Read the model definition and answer for the solid it produces. Units are mm, in the model's axes. Coordinates: 2 decimals unless noted, no trailing zeros. Order: outer loops, then holes, each group sorted by start corner. A loop starts at its lowest first (then second) coordinate and runs counter-clockwise, first axis right, second up. Notation, with made-up numbers: M 66.5,-6.5 L 112.5,-6.5 A15 cw 112.5,15.5 Z; hole C -20.75,14.5 d6. An arc over 180 degrees is marked long. Write each question's results on one line, items separated by ' | '.
```python
from build123d import *

# Parameters (mm, degrees)
SKETCH1_W           = 10
SKETCH1_H           = 24.4
SKETCH1_R           = 3
BOSS_EXTRUDE1_DEPTH = 10
FILLET1_R           = 2


with BuildPart() as part:
    # Sketch1 → Boss-Extrude1 (new body)
    with BuildSketch(Plane(origin=(0, 0, 0), x_dir=(1, 0, 0), z_dir=(0, 1, 0))):
        Rectangle(SKETCH1_W, SKETCH1_H)
        with Locations(Location((0, 0, 0), (0, 0, 270))):
            Circle(SKETCH1_R, mode=Mode.SUBTRACT)
    extrude(amount=BOSS_EXTRUDE1_DEPTH)

    # Fillet1
    fillet1_edges = [part.edges().sort_by_distance(p)[0] for p in [
        (-5, 10, 0),
        (5, 10, 0),
    ]]
    fillet(fillet1_edges, radius=FILLET1_R - 0.0001)  # a hair under: the kernel refuses the full size


solid = part.part
```
(1) The mould has two halves that part along X. Classify faces 1 (the cylindrical face through (4.43, 9.4, -0.17)), 2 (the cylindrical face through (0.9, 4.93, 2.86)), 3 (the cylindrical face through (-4.43, 9.4, -0.17)), 4 (the flat face through (-1, 10, -3)): pulls with the +X half, pulls with the -X half, needs draft (parallel to the pull), parting line crosses it, or undercut.
Conclusion:
face 1: pulls with the +X half | face 2: undercut | face 3: pulls with the -X half | face 4: needs draft
(2) Given pin 1 (1.5 mm diameter, centred on x = 0.5, z = 7, fed in from -Y); pin 2 (1.5 mm diameter, centred on x = -1, z = 0.5, fed in from -Y), each flat-ended and moving along its own axis, determine where each tip first touches the part or whether it passes through.
Conclusion:
pin 1: y = 0 | pin 2: through
(3) Straight lines are drawn through the part: line 1 (X direction, y = 4.75, z = 0); line 2 (Z direction, x = 0.75, y = 7.5); line 3 (X direction, y = 7, z = -0.75). For each, find the intervals that lie inside material, in ascending order.
Conclusion:
line 1: -5 to -3, 3 to 5 | line 2: -12.2 to -2.9, 2.9 to 12.2 | line 3: -5 to -2.9, 2.9 to 5
(4) The part is cut by section D-D, the plane z = -10.5. Write down the section's boundary in (x, y).
Conclusion:
outline: M -5,0 L 5,0 L 5,8 A2 ccw 3,10 L -3,10 A2 ccw -5,8 Z
(5) The part is cut by section B-B, the plane x = 0. Write down the section's boundary in (y, z).
Conclusion:
outline: M 0,-12.2 L 10,-12.2 L 10,-3 L 0,-3 Z; M 0,3 L 10,3 L 10,12.2 L 0,12.2 Z
(6) The part is cut by section C-C, the plane y = 5.25. Write down the section's boundary in (x, z).
Conclusion:
outline: M -5,-12.2 L 5,-12.2 L 5,12.2 L -5,12.2 Z; hole C 0,0 d6
